from build123d import *

# Parameters (mm, degrees)
SKETCH_1_R               = 14
EXTRUDE_1_DEPTH          = 4
CUT_EXTRUDE_1_DEPTH      = 4
PATTERN_CIRCULAR_1_COUNT = 26
CUT_EXTRUDE_2_REACH      = 6
SKETCH_5_R               = 3.6
SKETCH_5_R_2             = 1.65


with BuildPart() as part:
    # 草圖1 → 填料-伸長1 (new body)
    with BuildSketch(Plane.XY):
        Circle(SKETCH_1_R)
    extrude(amount=EXTRUDE_1_DEPTH)

    # 草圖4 → 除料-伸長1 (cut)
    with BuildSketch(Plane.XY.offset(4)):
        with BuildLine():
            ThreePointArc((-1.421594657, 13.927636865), (0, 14), (1.421594657, 13.927636865))
            ThreePointArc((1.421594657, 13.927636865), (0.822322703, 12.888806427), (0.476978653, 11.74031479))
            ThreePointArc((0.476978653, 11.74031479), (0, 11.75), (-0.476978653, 11.74031479))
            ThreePointArc((-0.476978653, 11.74031479), (-0.822322703, 12.888806427), (-1.421594657, 13.927636865))
        make_face()
    cut_extrude_1 = extrude(amount=-CUT_EXTRUDE_1_DEPTH, mode=Mode.SUBTRACT)

    # 環狀複製排列1: 除料-伸長1 ×26 about axis
    pattern_circular_1_axis = Axis((0, 0, 0), (0, 0, 1))
    for i in range(1, PATTERN_CIRCULAR_1_COUNT):
        add(cut_extrude_1.rotate(pattern_circular_1_axis, i * 360 / PATTERN_CIRCULAR_1_COUNT), mode=Mode.SUBTRACT)

    # 草圖5 → 除料-伸長2 (cut, up to next)
    with BuildSketch(Plane.XY.offset(4), mode=Mode.PRIVATE) as cut_extrude_2_sk1:
        Circle(SKETCH_5_R)
    cut_extrude_2_tool1 = extrude(cut_extrude_2_sk1.sketch, amount=-CUT_EXTRUDE_2_REACH, mode=Mode.PRIVATE) & part.part
    add(cut_extrude_2_tool1.solids().sort_by_distance((0, 0, 4))[0], mode=Mode.SUBTRACT)
    # 草圖5 → 除料-伸長2 (cut, up to next)
    with BuildSketch(Plane.XY.offset(4), mode=Mode.PRIVATE) as cut_extrude_2_sk2:
        with Locations((0, 8)):
            Circle(SKETCH_5_R_2)
    cut_extrude_2_tool2 = extrude(cut_extrude_2_sk2.sketch, amount=-CUT_EXTRUDE_2_REACH, mode=Mode.PRIVATE) & part.part
    add(cut_extrude_2_tool2.solids().sort_by_distance((0, 8, 4))[0], mode=Mode.SUBTRACT)
    # 草圖5 → 除料-伸長2 (cut, up to next)
    with BuildSketch(Plane.XY.offset(4), mode=Mode.PRIVATE) as cut_extrude_2_sk3:
        with Locations((8, 0)):
            Circle(SKETCH_5_R_2)
    cut_extrude_2_tool3 = extrude(cut_extrude_2_sk3.sketch, amount=-CUT_EXTRUDE_2_REACH, mode=Mode.PRIVATE) & part.part
    add(cut_extrude_2_tool3.solids().sort_by_distance((8, 0, 4))[0], mode=Mode.SUBTRACT)
    # 草圖5 → 除料-伸長2 (cut, up to next)
    with BuildSketch(Plane.XY.offset(4), mode=Mode.PRIVATE) as cut_extrude_2_sk4:
        with Locations((0, -8)):
            Circle(SKETCH_5_R_2)
    cut_extrude_2_tool4 = extrude(cut_extrude_2_sk4.sketch, amount=-CUT_EXTRUDE_2_REACH, mode=Mode.PRIVATE) & part.part
    add(cut_extrude_2_tool4.solids().sort_by_distance((0, -8, 4))[0], mode=Mode.SUBTRACT)
    # 草圖5 → 除料-伸長2 (cut, up to next)
    with BuildSketch(Plane.XY.offset(4), mode=Mode.PRIVATE) as cut_extrude_2_sk5:
        with Locations((-8, 0)):
            Circle(SKETCH_5_R_2)
    cut_extrude_2_tool5 = extrude(cut_extrude_2_sk5.sketch, amount=-CUT_EXTRUDE_2_REACH, mode=Mode.PRIVATE) & part.part
    add(cut_extrude_2_tool5.solids().sort_by_distance((-8, 0, 4))[0], mode=Mode.SUBTRACT)


solid = part.part
Can you work these out from the model? Positions are in its coordinate system, mm. A direction names the side the tool comes from. Coordinates: 2 decimals unless noted, no trailing zeros. Order: outer loops, then holes, each group sorted by start corner. A loop starts at its lowest first (then second) coordinate and runs counter-clockwise, first axis right, second up. Notation, with made-up numbers: (-16.5, 69) - (35.5, 69) arc R8 ccw to (35.5, 81) - close; hole circle Ø10 at (-13.75, -31.5). An arc over 180 degrees is marked (long way). Answer as a JSON object with one key per item and string values. Group by question number.
Q1. I need wall thicknesses on line 1 (Y direction, x = 0, z = 1.7); line 2 (Y direction, x = -10, z = 2.85); line 3 (Y direction, x = -10.5, z = 1.25). Which ranges of each line are inside material? Lowest first, please. Write a range as from..to.
Q2. Imagine slicing it at C-C (z = 3.25). Give the number of separate pieces and of enclosed holes in the cut face, and give its area (3 significant figures).
Q3. On a 3-axis mill with a long thin cutter (end or side, diameter ignored), from which of +Z, -Z, +X, -X, +Y, -Y can I reach the whole of each face in a straight line? I mean faces 4 (the face through (-11.75, -5.33, 2.03)), 5 (the face through (-11.06, 6.64, 2.03)), 6 (the face through (6.73, 11.04, 2.03)), 7 (the face through (11.665, 1.41, 2.028)). Say none if no direction works.
Q4. We'd pull the mould along X, two halves only. Please class faces 1 (the face through (-2.283, 12.728, 2.028)), 2 (the face through (-12.71, 2.38, 2.03)), 3 (the face through (12.68, 2.36, 2.03)): +X half, -X half, draft (parallel to the pull), parting line (faces both ways), or undercut.
Q5. Imagine slicing it at B-B (x = -1). Please give me the cut outline in (y, z).
Q6. Imagine slicing it at A-A (y = 8). Please give me the cut outline in (x, z), and give its area (3 significant figures).
Determined:
{
 "1": {"line 1": "y = -11.75..-9.65, -6.35..-3.6, 3.6..6.35, 9.65..11.75", "line 2": "y = -9.41..-7.79, -6.31..6.31, 7.79..9.41", "line 3": "y = -9.26..-8.68, -6.5..6.5, 8.68..9.26"},
 "2": {"separate pieces": "1", "enclosed holes": "5", "area": "441 mm2"},
 "3": {"face 4": "+Z, -Z, -X", "face 5": "+Z, -Z", "face 6": "+Z, -Z, +Y", "face 7": "+Z, -Z, +X"},
 "4": {"face 1": "undercut", "face 2": "-X half", "face 3": "+X half"},
 "5": {"outline": "(-13.26, 0) - (-9.31, 0) - (-9.31, 4) - (-13.26, 4) - close; (-6.69, 0) - (-3.46, 0) - (-3.46, 4) - (-6.69, 4) - close; (3.46, 0) - (6.69, 0) - (6.69, 4) - (3.46, 4) - close; (9.31, 0) - (13.26, 0) - (13.26, 4) - (9.31, 4) - close"},
 "6": {"outline": "(-10.14, 0) - (-1.65, 0) - (-1.65, 4) - (-10.14, 4) - close; (1.65, 0) - (10.14, 0) - (10.14, 4) - (1.65, 4) - close", "area": "67.9 mm2"}
}
